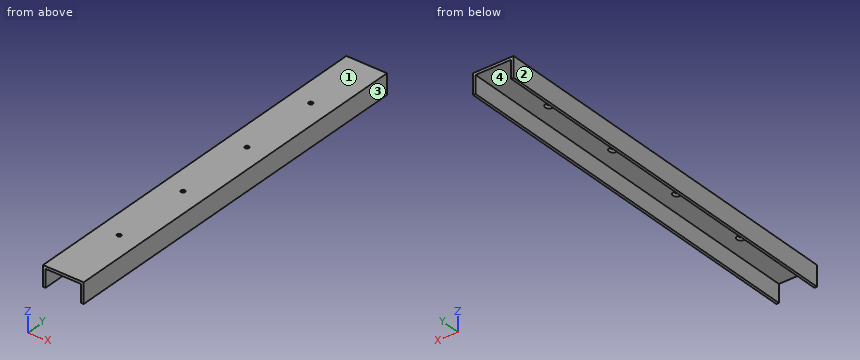
from build123d import *

# Parameters (mm, degrees)
BOSS_EXTRUDE1_DEPTH = 241.3
LPATTERN1_COUNT     = 4
LPATTERN1_PITCH     = 101.6


with BuildPart() as part:
    # Sketch1 → Boss-Extrude1 (new, symmetric)
    with BuildSketch(Plane(origin=(0, 0, 0), x_dir=(1, 0, 0), z_dir=(0, 1, 0))):
        Polygon((-25.4, 12.7), (-25.4, -12.7), (25.4, -12.7), (25.4, 12.7), (22.225, 12.7), (22.225, -9.525), (-22.225, -9.525), (-22.225, 12.7), align=None)
    extrude(amount=BOSS_EXTRUDE1_DEPTH, both=True)

    # Sketch2 → CSK for #10 Flat Head Machine Screw (100)1 (revolve, cut)
    with BuildSketch(Plane(origin=(0, -152.4, 9.525), x_dir=(0, 1, 0), z_dir=(1, 0, 0))):
        Polygon((0, 0), (0, 3.175), (2.5527, 3.175), (2.5527, 1.960808018), (4.8895, 0), align=None)
    csk_for_10_flat_head_machine_screw_100 = revolve(axis=Axis((0, -152.4, 3.175), (0, 0, 1)), mode=Mode.SUBTRACT)

    # LPattern1: CSK for #10 Flat Head Machine Screw (100)1 ×4
    with Locations(*[(0, i * LPATTERN1_PITCH, 0) for i in range(1, LPATTERN1_COUNT)]):
        add(csk_for_10_flat_head_machine_screw_100, mode=Mode.SUBTRACT)


solid = part.part
Input: part model. Units: mm. Frame: model coordinates. Face numbers are marked on the shaded views. Give positions to 0.01 mm unless a question says otherwise; leave off trailing zeros. Write each loop counter-clockwise with the first axis right and the second up, starting at its lowest first coordinate (ties: lowest second). Pieces come first, ordered by that corner, then holes. Notation, with made-up numbers: (62.25, -15) -> (72.25, -15) arc R15 cw to (72.25, -9) -> close; hole circle Ø2 at (80, -22). An arc over 180 degrees is marked (long way). Use one line per item in the form item = value. Start each with the question number.
1) Draft query along X for the marked faces 1, 2, 3 and 4. Return one class per face: pulls with the +X half, pulls with the -X half, needs draft (parallel to the pull), parting line crosses it, or undercut.
2) Ray query, probe 1 along Y at (x, z) = (0, 12.3); probe 2 along X at (y, z) = (113, 8.5) (3 decimals); probe 3 along X at (y, z) = (-152.4, 12.05). Return the intervals inside material, ascending. Write a range as from..to.
3) Section query A-A on z = -5. Return the cut outline in (x, y) (3 decimals), then the cut area to 3 significant figures.
4) Section query B-B on y = 67. Return the cut outline in (x, z) (3 decimals), then the cut area to 3 significant figures.
5) Pin query (flat end, axial travel): pin 1 (4 mm diameter, centred on x = 12.5, y = -79, fed in from -Z) (3 decimals); pin 2 (4 mm diameter, centred on x = 3.5, z = 6.5, fed in from -Y); pin 3 (8 mm diameter, centred on x = 0, y = 152.4, fed in from -Z); pin 4 (6.5 mm diameter, centred on x = 0, y = 50.8, fed in from -Z). Return the tip coordinate at first contact, or that it passes through.
6) Section query C-C on x = -15.5. Return the cut outline in (y, z) (3 decimals).
Outcome:
q1.face_1 = needs draft
q1.face_2 = pulls with the -X half
q1.face_3 = pulls with the +X half
q1.face_4 = undercut
q2.probe_1 = -241.3..-154.95, -149.85..-53.35, -48.25..48.25, 53.35..149.85, 154.95..241.3
q2.probe_2 = -25.4..-22.225, 22.225..25.4
q2.probe_3 = -25.4..-2.55, 2.55..25.4
q3.outline = (-25.4, -241.3) -> (-22.225, -241.3) -> (-22.225, 241.3) -> (-25.4, 241.3) -> close; (22.225, -241.3) -> (25.4, -241.3) -> (25.4, 241.3) -> (22.225, 241.3) -> close
q3.area = 3,060 mm^2
q4.outline = (-25.4, -12.7) -> (-22.225, -12.7) -> (-22.225, 9.525) -> (22.225, 9.525) -> (22.225, -12.7) -> (25.4, -12.7) -> (25.4, 12.7) -> (-25.4, 12.7) -> close
q4.area = 302 mm^2
q5.pin_1 = 9.525
q5.pin_2 = through
q5.pin_3 = 10.27
q5.pin_4 = 10.9
q6.outline = (-241.3, 9.525) -> (241.3, 9.525) -> (241.3, 12.7) -> (-241.3, 12.7) -> close
